The listing builds one solid part. Answer for the finished solid, in the listing's coordinates (mm). Face numbers are marked on the shaded views. A direction names the side the tool comes from. Round coordinates to 2 decimals unless told otherwise and drop trailing zeros. Order: outer loops, then holes, each group sorted by start corner. A loop starts at its lowest first (then second) coordinate and runs counter-clockwise, first axis right, second up. Notation, with made-up numbers: (67.5, -18) - (110.5, -18) arc R20 ccw to (110.5, 15) - close; hole circle Ø10 at (78.5, 59.5). An arc over 180 degrees is marked (long way). Use CSV: the item, a comma, the result in double quotes. Start each with the question number.
Item 1: Find section C-C, the plane y = -2.5. Give the vertices of the cut face in (x, z), plus the area to 3 significant figures.
Item 2: Find section B-B, the plane z = -1.5. Give the vertices of the cut face in (x, y) (3 decimals), plus the area to 3 significant figures.
Item 3: Straight lines are drawn through the part: line 1 along Y through (x, z) = (38, 2); line 2 along X through (y, z) = (-18.5, -7.5); line 3 along Y through (x, z) = (38.1, 23.25). For each, find the intervals that lie inside material, in ascending order. Write a range as [from, to].
Item 4: Determine the mould class of the marked faces 4, 5 and 6 for opening direction X: +X half, -X half, draft (parallel to the pull), parting line (faces both ways), or undercut.
Item 5: For the marked faces 1, 2 and 3, determine the directions among +Z, -Z, +X, -X, +Y, -Y from which every point of the face is accessible in a straight line to the end or side of a thin tool.
Item 6: Find section D-D, the plane y = -20. Give the vertices of the cut face in (x, z), plus the area to 3 significant figures.
Item 7: Find section A-A, the plane y = -13.5. Give the vertices of the cut face in (x, z).
Item 8: Flat-ended cylindrical pins translate along their axes: P1, Ø4, axis at x = 33.5, z = 19.5, coming from the +Y side; P2, Ø6, axis at x = 9.5, y = -12.5, coming from the +Z side. Find the tip coordinate at first contact, or state that the pin passes through.
```python
from build123d import *

# Parameters (mm, degrees)
F0_W      = 76.2
F0_H      = 12.7
F1_DEPTH  = 38.1
F2_R      = 9.525
F3_DEPTH  = 6.35
F3_FACE_R = 9.525
F4_DEPTH  = 12.701
F5_R      = 19.05
F5_R_2    = 9.525
F6_DEPTH  = 19.05
F7_R      = 19.05
F7_R_2    = 12.7
F8_DEPTH  = 6.35
F9_R      = 19.05
F9_R_2    = 9.525
F10_DEPTH = 6.35


with BuildPart() as f1:
    # F0 (on Front) → F1 (new body)
    with BuildSketch(Plane.XZ):
        with Locations((38.1, 6.35)):
            Rectangle(F0_W, F0_H)
    extrude(amount=F1_DEPTH)

    # F2 (on face) → F3 (join)
    with BuildSketch(Plane.XY.offset(12.7)):
        with BuildLine():
            ThreePointArc((38.1, -38.1), (51.570384, -32.520384), (57.15, -19.05))
            ThreePointArc((57.15, -19.05), (51.570384, -5.579616), (38.1, 0))
            ThreePointArc((38.1, 0), (19.05, -19.05), (38.1, -38.1))
        make_face()
        with Locations((38.1, -19.05)):
            Circle(F2_R, mode=Mode.SUBTRACT)
    extrude(amount=F3_DEPTH)

    # F3_face (on face) → F4 (cut, through all)
    with BuildSketch(Plane(origin=(38.1, -19.05, 12.7), x_dir=(1, 0, 0), z_dir=(0, 0, 1))):
        Circle(F3_FACE_R)
    extrude(amount=-F4_DEPTH, mode=Mode.SUBTRACT)

    # F5 (on face) → F6 (join)
    with BuildSketch(Plane(origin=(0, 0, 0), x_dir=(1, 0, 0), z_dir=(0, 0, -1))):
        with Locations((38.1, 19.05)):
            Circle(F5_R)
        with Locations((38.1, 19.05)):
            Circle(F5_R_2, mode=Mode.SUBTRACT)
    extrude(amount=F6_DEPTH)

    # F7 (on face) → F8 (join)
    with BuildSketch(Plane.XY.offset(19.05)):
        with Locations((38.1, -19.05)):
            Circle(F7_R)
        with Locations((38.1, -19.05)):
            Circle(F7_R_2, mode=Mode.SUBTRACT)
    extrude(amount=F8_DEPTH)

    # F9 (on face) → F10 (join)
    with BuildSketch(Plane.XY.offset(25.4)):
        with Locations((38.1, -19.05)):
            Circle(F9_R)
        with Locations((38.1, -19.05)):
            Circle(F9_R_2, mode=Mode.SUBTRACT)
    extrude(amount=F10_DEPTH)


solid = f1.part
```
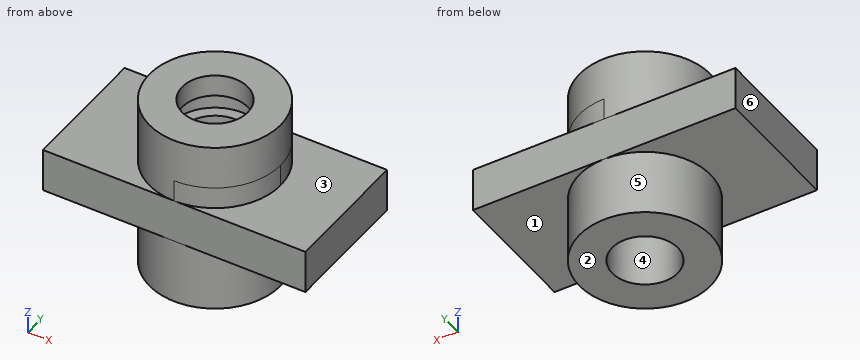
Worked out:
1,outline,"(0, 0) - (28.67, 0) - (28.67, -19.05) - (47.53, -19.05) - (47.53, 0) - (76.2, 0) - (76.2, 12.7) - (47.53, 12.7) - (47.53, 31.75) - (28.67, 31.75) - (28.67, 12.7) - (0, 12.7) - close"
1,area,"1,690 mm²"
2,outline,"circle Ø38.1 at (38.1, -19.05); hole circle Ø19.05 at (38.1, -19.05)"
2,area,"855 mm²"
3,line 1,"y = [-38.1, -28.57], [-9.53, 0]"
3,line 2,"x = [19.06, 28.59], [47.61, 57.14]"
3,line 3,"y = [-38.1, -31.75], [-6.35, 0]"
4,face 4,"undercut"
4,face 5,"parting line"
4,face 6,"-X half"
5,face 1,"-Z, +X"
5,face 2,"-Z, +X, -X, +Y, -Y"
5,face 3,"+Z, +X"
6,outline,"(0, 0) - (19.07, 0) - (19.07, -19.05) - (28.62, -19.05) - (28.62, 19.05) - (25.44, 19.05) - (25.44, 25.4) - (28.62, 25.4) - (28.62, 31.75) - (19.07, 31.75) - (19.07, 12.7) - (0, 12.7) - close; (47.58, -19.05) - (57.13, -19.05) - (57.13, 0) - (76.2, 0) - (76.2, 12.7) - (57.13, 12.7) - (57.13, 31.75) - (47.58, 31.75) - (47.58, 25.4) - (50.76, 25.4) - (50.76, 19.05) - (47.58, 19.05) - close"
6,area,"1,410 mm²"
7,outline,"(0, 0) - (19.88, 0) - (19.88, -19.05) - (30.36, -19.05) - (30.36, 19.05) - (26.68, 19.05) - (26.68, 25.4) - (30.36, 25.4) - (30.36, 31.75) - (19.88, 31.75) - (19.88, 12.7) - (0, 12.7) - close; (45.84, -19.05) - (56.32, -19.05) - (56.32, 0) - (76.2, 0) - (76.2, 12.7) - (56.32, 12.7) - (56.32, 31.75) - (45.84, 31.75) - (45.84, 25.4) - (49.52, 25.4) - (49.52, 19.05) - (45.84, 19.05) - close"
8,P1,"stops at y = -0.18"
8,P2,"stops at z = 12.7"
